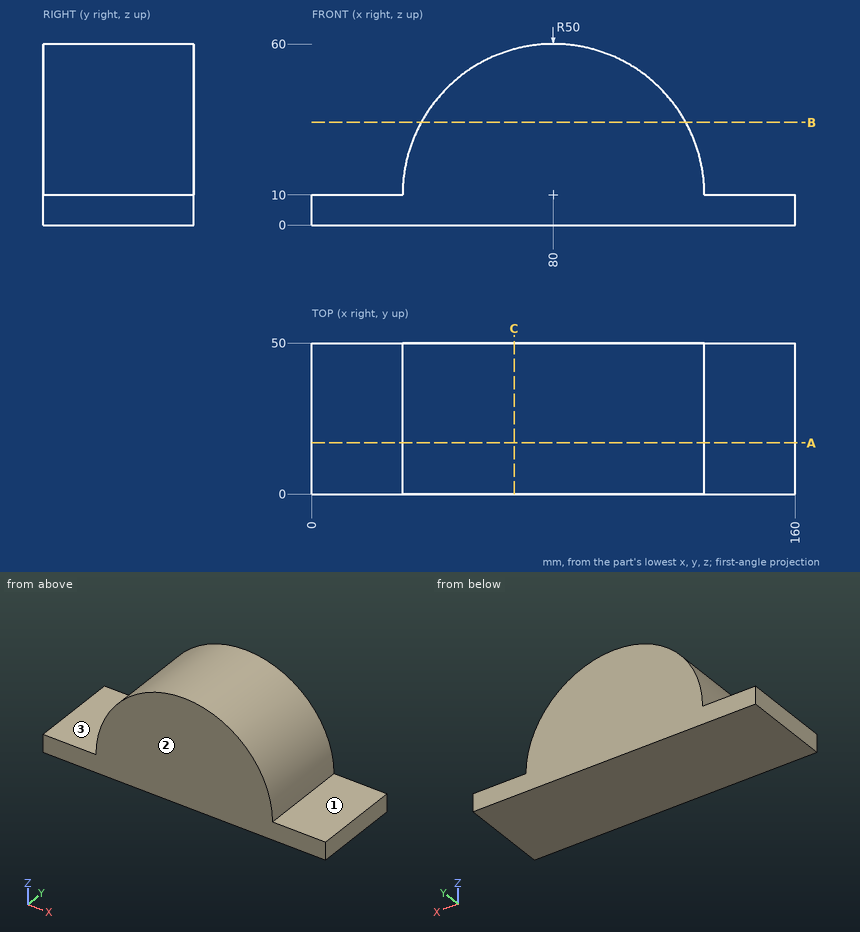
Drawing for the job (mm, zero at the part's lowest x, y, z). A direction names the side the tool comes from. Coordinates: 2 decimals unless noted, no trailing zeros. Write each loop counter-clockwise with the first axis right and the second up, starting at its lowest first coordinate (ties: lowest second). Pieces come first, ordered by that corner, then holes. Notation, with made-up numbers: (39.25, 30.5) -> (77.25, 30.5) arc R26 cw to (77.25, 68.5) -> close; hole circle Ø9 at (32.25, 8.5). An arc over 180 degrees is marked (long way). One line per item, written item: value. Start each with the question number.
1) Which spindle directions (+Z, -Z, +X, -X, +Y, -Y) get a long thin tool onto all of the face, cutting with end or side? Do the marked faces 1, 2 and 3. Say none if no direction does.
2) Probe probe 1 along Z at (x, y) = (141.5, 21.5); probe 2 along X at (y, z) = (19, 11.5); probe 3 along Z at (x, y) = (98.5, 5). List the from-to ranges inside material, lowest first.
3) Slice it at B-B on z = 34. Write the cut outline in (x, y), then the cut area to 3 significant figures.
4) Slice it at A-A on y = 17. Write the cut outline in (x, z), then the cut area to 3 significant figures.
5) Slice it at C-C on x = 67. Write the cut outline in (y, z).
6) Flat gauge pins, fed straight in: pin 1 Ø1.5 at (x, y) = (98.5, 5.5) entering from -Z; pin 2 Ø4 at (y, z) = (33.5, 35) entering from -X; pin 3 Ø10 at (x, y) = (92.5, 26) entering from +Z; pin 4 Ø5 at (x, y) = (87.5, 15) entering from +Z. Where does each tip first touch, or does it go through?
Answers follow:
1. face 1: +Z, +X, +Y, -Y
1. face 2: +Z, -Z, +X, -X, -Y
1. face 3: +Z, -X, +Y, -Y
2. probe 1: 0 to 10
2. probe 2: 30.02 to 129.98
2. probe 3: 0 to 56.45
3. outline: (36.14, 0) -> (123.86, 0) -> (123.86, 50) -> (36.14, 50) -> close
3. area: 4,390 mm2
4. outline: (0, 0) -> (160, 0) -> (160, 10) -> (130, 10) arc R50 ccw to (30, 10) -> (0, 10) -> close
4. area: 5,530 mm2
5. outline: (0, 0) -> (50, 0) -> (50, 58.28) -> (0, 58.28) -> close
6. pin 1: z = 0
6. pin 2: x = 35.6
6. pin 3: z = 59.43
6. pin 4: z = 59.75
